Verification items for the finished model (mm, model axes). A direction names the side the tool comes from. Coordinates: 2 decimals unless noted, no trailing zeros. Order: outer loops, then holes, each group sorted by start corner. A loop starts at its lowest first (then second) coordinate and runs counter-clockwise, first axis right, second up. Notation, with made-up numbers: M -5.5,-15.5 L 33.5,-15.5 A25 ccw 33.5,-3.5 Z; hole C 89.5,78.5 d11. An arc over 180 degrees is marked long. Return JSON: item names as keys, results as strings. Group by question number.
Q1. Thickness scan on probe 1 along Y at (x, z) = (-143.85, -109); probe 2 along Z at (x, y) = (139, 199.25); probe 3 along Z at (x, y) = (-81, 82). Record the ranges inside material, lowest first.
Q2. Mould release check, pull along X, two halves, no side actions. Record for faces 3 (the face through (-143, 101, -108)), 4 (the face through (139, 200, 8)), 5 (the face through (-145, 101, 109)): pulls with the +X half, pulls with the -X half, needs draft (parallel to the pull), parting line crosses it, or undercut.
Q3. Access from +Z, -Z, +X, -X, +Y, -Y to the whole of each face (thin tool, end or side, straight path). Record for faces 1 (the face through (-2, 101, -113)), 2 (the face through (-145, 101, -109)).
Q4. Section check B-B, the plane y = 110.5. Enter the section's corners in (x, z).
Q5. Section check A-A, the plane x = -51.5. Enter the section's corners in (y, z).
Q6. Section check C-C, the plane z = -67.5. Enter the section's corners in (x, y), then the cut area to 3 significant figures.
Q7. Go/stop test with flat-tipped pins: pin 1 Ø10 at (y, z) = (81, 29) entering from -X; pin 2 Ø1.6 at (x, z) = (139, 104) entering from -Y; pin 3 Ø1.6 at (y, z) = (198.5, -21.5) entering from -X; pin 4 Ø5 at (x, z) = (138.5, 10.5) entering from -Y. Record where each tip stops, or that it passes through.
from build123d import *

# Parameters (mm, degrees)
SKETCH_1_W          = 290
SKETCH_1_H          = 230
EXTRUDE_1_DEPTH     = 200
SKETCH_2_W          = 286
SKETCH_2_H          = 226
CUT_EXTRUDE_1_DEPTH = 200
SKETCH_3_W          = 226
SKETCH_3_H          = 200
CUT_EXTRUDE_2_DEPTH = 2
SKETCH_5_W          = 10
SKETCH_5_H          = 220
EXTRUDE_2_DEPTH     = 2
SKETCH_6_R          = 1.6
CUT_EXTRUDE_3_DEPTH = 2
SKETCH_7_R          = 1.350525158
CUT_EXTRUDE_4_DEPTH = 2
SKETCH_8_W          = 10
SKETCH_8_H          = 200
EXTRUDE_3_DEPTH     = 2
SKETCH_9_R          = 1.6
CUT_EXTRUDE_5_DEPTH = 2
SKETCH_10_R         = 1.6
CUT_EXTRUDE_6_DEPTH = 2
SKETCH_11_W         = 10
SKETCH_11_H         = 200
EXTRUDE_4_DEPTH     = 2
SKETCH_12_R         = 1.6
CUT_EXTRUDE_7_DEPTH = 2
SKETCH_13_R         = 1.6
CUT_EXTRUDE_8_DEPTH = 2


with BuildPart() as part:
    # 草图1 → 凸台-拉伸1 (new body)
    with BuildSketch(Plane(origin=(0, 0, 0), x_dir=(1, 0, 0), z_dir=(0, 1, 0))):
        Rectangle(SKETCH_1_W, SKETCH_1_H)
    extrude(amount=EXTRUDE_1_DEPTH)

    # 草图2 → 切除-拉伸1 (cut)
    with BuildSketch(Plane(origin=(0, 200, 0), x_dir=(1, 0, 0), z_dir=(0, 1, 0))):
        Rectangle(SKETCH_2_W, SKETCH_2_H)
    extrude(amount=-CUT_EXTRUDE_1_DEPTH, mode=Mode.SUBTRACT)

    # 草图3 → 切除-拉伸2 (cut)
    with BuildSketch(Plane.ZY.offset(145)):
        with Locations((0, 100)):
            Rectangle(SKETCH_3_W, SKETCH_3_H)
    extrude(amount=-CUT_EXTRUDE_2_DEPTH, mode=Mode.SUBTRACT)

    # 草图5 → 凸台-拉伸2 (add)
    with BuildSketch(Plane(origin=(0, 200, 0), x_dir=(1, 0, 0), z_dir=(0, 1, 0))):
        with Locations((138, 0)):
            Rectangle(SKETCH_5_W, SKETCH_5_H)
    extrude(amount=-EXTRUDE_2_DEPTH)

    # 草图6 → 切除-拉伸3 (cut)
    with BuildSketch(Plane(origin=(0, 200, 0), x_dir=(1, 0, 0), z_dir=(0, 1, 0))):
        with Locations(Location((138.825354176, 104, 0), (0, 0, 270))):
            Circle(SKETCH_6_R)
    extrude(amount=-CUT_EXTRUDE_3_DEPTH, mode=Mode.SUBTRACT)

    # 草图7 → 切除-拉伸4 (cut)
    with BuildSketch(Plane(origin=(0, 200, 0), x_dir=(1, 0, 0), z_dir=(0, 1, 0))):
        with Locations(Location((139, -104, 0), (0, 0, 270))):
            Circle(SKETCH_7_R)
    extrude(amount=-CUT_EXTRUDE_4_DEPTH, mode=Mode.SUBTRACT)

    # 草图8 → 凸台-拉伸3 (add)
    with BuildSketch(Plane.ZY.offset(145)):
        with Locations((108, 100)):
            Rectangle(SKETCH_8_W, SKETCH_8_H)
    extrude(amount=-EXTRUDE_3_DEPTH)

    # 草图9 → 切除-拉伸5 (cut)
    with BuildSketch(Plane.ZY.offset(145)):
        with Locations((109, 194)):
            Circle(SKETCH_9_R)
    extrude(amount=-CUT_EXTRUDE_5_DEPTH, mode=Mode.SUBTRACT)

    # 草图10 → 切除-拉伸6 (cut)
    with BuildSketch(Plane.ZY.offset(145)):
        with Locations((109, 6)):
            Circle(SKETCH_10_R)
    extrude(amount=-CUT_EXTRUDE_6_DEPTH, mode=Mode.SUBTRACT)

    # 草图11 → 凸台-拉伸4 (add)
    with BuildSketch(Plane.ZY.offset(145)):
        with Locations((-108, 100)):
            Rectangle(SKETCH_11_W, SKETCH_11_H)
    extrude(amount=-EXTRUDE_4_DEPTH)

    # 草图12 → 切除-拉伸7 (cut)
    with BuildSketch(Plane.ZY.offset(145)):
        with Locations((-109, 194)):
            Circle(SKETCH_12_R)
    extrude(amount=-CUT_EXTRUDE_7_DEPTH, mode=Mode.SUBTRACT)

    # 草图13 → 切除-拉伸8 (cut)
    with BuildSketch(Plane.ZY.offset(145)):
        with Locations((-109, 6)):
            Circle(SKETCH_13_R)
    extrude(amount=-CUT_EXTRUDE_8_DEPTH, mode=Mode.SUBTRACT)


solid = part.part
Numbers:
{
 "1": {"probe 1": "y = 0 to 4.4, 7.6 to 192.4, 195.6 to 200", "probe 2": "z = -115 to -113, -110 to -105.59, -102.41 to 102.65, 105.35 to 110, 113 to 115", "probe 3": "z = -115 to -113, 113 to 115"},
 "2": {"face 3": "undercut", "face 4": "needs draft", "face 5": "pulls with the -X half"},
 "3": {"face 1": "+Y, -Y", "face 2": "+Z, -Z, -X, +Y, -Y"},
 "4": {"outline": "M -145,-115 L 145,-115 L 145,115 L -145,115 L -145,103 L -143,103 L -143,113 L 143,113 L 143,-113 L -143,-113 L -143,-103 L -145,-103 Z"},
 "5": {"outline": "M 0,-115 L 200,-115 L 200,-113 L 0,-113 Z; M 0,113 L 200,113 L 200,115 L 0,115 Z"},
 "6": {"outline": "M 133,198 L 143,198 L 143,0 L 145,0 L 145,200 L 133,200 Z", "area": "420 mm2"},
 "7": {"pin 1": "stops at x = 143", "pin 2": "passes through", "pin 3": "stops at x = 133", "pin 4": "stops at y = 198"}
}
